Work out the finished part from the listing and answer in its coordinate system (mm). Give positions to 0.01 mm unless a question says otherwise; leave off trailing zeros. Loops run counter-clockwise (first coordinate to the right, second up) from the corner with the lowest first, then second, coordinate; pieces in that order, holes last. Notation, with made-up numbers: (38, 46) - (67, 46) arc R18 cw to (67, 68) - close; hole circle Ø5 at (37.5, 73). An arc over 180 degrees is marked (long way). Use CSV: the item, a comma, the result in double quotes.
from build123d import *

# Parameters (mm, degrees)
SKETCH1_R                                       = 2.4892
SKETCH1_R_2                                     = 2.5527
BOSS_EXTRUDE1_DEPTH                             = 3.175
FILLET1_R                                       = 4.7625
CSK_FOR_10_FLAT_HEAD_MACHINE_SCREW1_D           = 5.1054
CSK_FOR_10_FLAT_HEAD_MACHINE_SCREW1_DEPTH       = 19.05
CSK_FOR_10_FLAT_HEAD_MACHINE_SCREW1_CSINK_D     = 9.779
CSK_FOR_10_FLAT_HEAD_MACHINE_SCREW1_CSINK_ANGLE = 82
CSK_FOR_10_FLAT_HEAD_MACHINE_SCREW1_TIP         = 1.533816902


with BuildPart() as part:
    # Sketch1 → Boss-Extrude1 (new body)
    with BuildSketch(Plane.XY):
        Polygon((-37.846, 23.8125), (-37.846, -21.2725), (45.72, -21.2725), (45.72, 0.3175), (-21.59, 0.3175), (-21.59, 23.8125), align=None)
        with Locations((-29.845, -11.1125)):
            Circle(SKETCH1_R, mode=Mode.SUBTRACT)
        with Locations((-7.62, -11.1125)):
            Circle(SKETCH1_R, mode=Mode.SUBTRACT)
        with Locations((1.905, -11.1125)):
            Circle(SKETCH1_R_2, mode=Mode.SUBTRACT)
        with Locations((27.305, -11.1125)):
            Circle(SKETCH1_R_2, mode=Mode.SUBTRACT)
        with Locations((-29.845, 1.5875)):
            Circle(SKETCH1_R, mode=Mode.SUBTRACT)
        with Locations((-29.845, 14.2875)):
            Circle(SKETCH1_R, mode=Mode.SUBTRACT)
        with Locations((-29.845, -11.1125)):
            Circle(SKETCH1_R)
    extrude(amount=BOSS_EXTRUDE1_DEPTH)

    # Fillet1
    fillet1_edges = [part.edges().sort_by_distance(p)[0] for p in [
        (-37.846, 23.8125, 1.5875),
        (-21.59, 23.8125, 1.5875),
        (-21.59, 0.3175, 1.5875),
        (45.72, 0.3175, 1.5875),
        (45.72, -21.2725, 1.5875),
        (-37.846, -21.2725, 1.5875),
    ]]
    fillet(fillet1_edges, radius=FILLET1_R)

    # CSK for #10 Flat Head Machine Screw1
    with Locations(Plane.XY.offset(3.175)):
        with Locations((27.305, -11.1125)):
            CounterSinkHole(CSK_FOR_10_FLAT_HEAD_MACHINE_SCREW1_D / 2, CSK_FOR_10_FLAT_HEAD_MACHINE_SCREW1_CSINK_D / 2, depth=CSK_FOR_10_FLAT_HEAD_MACHINE_SCREW1_DEPTH, counter_sink_angle=CSK_FOR_10_FLAT_HEAD_MACHINE_SCREW1_CSINK_ANGLE)
            with Locations((0, 0, -(CSK_FOR_10_FLAT_HEAD_MACHINE_SCREW1_DEPTH + CSK_FOR_10_FLAT_HEAD_MACHINE_SCREW1_TIP / 2))):  # 118° drill point
                Cone(0, CSK_FOR_10_FLAT_HEAD_MACHINE_SCREW1_D / 2, CSK_FOR_10_FLAT_HEAD_MACHINE_SCREW1_TIP, mode=Mode.SUBTRACT)


solid = part.part
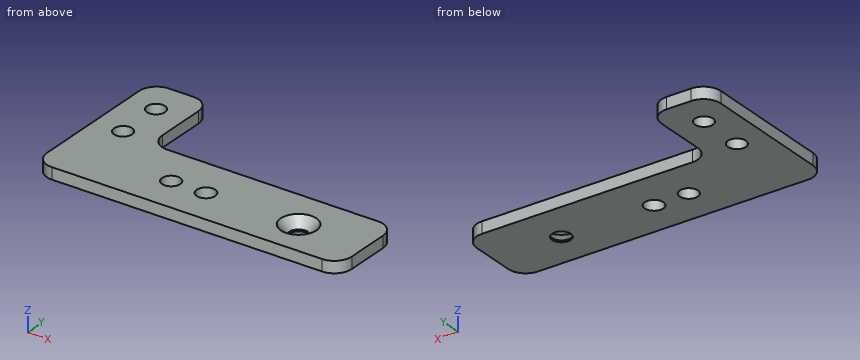
Item 1: Find the intervals of material crossed by line 1 (Y direction, x = 26, z = 0.8); line 2 (Y direction, x = -28, z = 0.6); line 3 (X direction, y = 9, z = 2.3), in increasing order.
Determined:
line 1,"y = -21.27 to -13.62, -8.61 to 0.32"
line 2,"y = -21.27 to -0.08, 3.26 to 12.62, 15.96 to 23.81"
line 3,"x = -37.85 to -21.59"
Item 2: A cutting plane is placed at C-C on x = -30.5. Determine the outline of the cut face in (y, z) (1 decimal), and give its area (3 significant figures).
Determined:
outline,"(-21.3, 0) - (-0.8, 0) - (-0.8, 3.2) - (-21.3, 3.2) - close; (4, 0) - (11.9, 0) - (11.9, 3.2) - (4, 3.2) - close; (16.7, 0) - (23.8, 0) - (23.8, 3.2) - (16.7, 3.2) - close"
area,"113 mm²"
Item 3: A cutting plane is placed at B-B on y = 2.5. Determine the outline of the cut face in (x, z) (3 decimals), and give its area (3 significant figures).
Determined:
outline,"(-37.846, 0) - (-32.161, 0) - (-32.161, 3.175) - (-37.846, 3.175) - close; (-27.529, 0) - (-20.831, 0) - (-20.831, 3.175) - (-27.529, 3.175) - close"
area,"39.3 mm²"
Item 4: A cutting plane is placed at A-A on x = -7.62. Determine the outline of the cut face in (y, z) (1 decimal), and give its area (3 significant figures).
Determined:
outline,"(-21.3, 0) - (-13.6, 0) - (-13.6, 3.2) - (-21.3, 3.2) - close; (-8.6, 0) - (0.3, 0) - (0.3, 3.2) - (-8.6, 3.2) - close"
area,"52.7 mm²"
Item 5: A cutting plane is placed at D-D on z = 2. State how many separate pieces and enclosed holes the cut face has, and give its area (3 significant figures).
Determined:
separate pieces,"1"
enclosed holes,"5"
area,"2,040 mm²"
Item 6: Given P1, Ø1, axis at y = 15, z = 2, coming from the +X side, flat-ended and moving along its own axis, determine where the tip first touches the part or whether it passes through.
Determined:
P1,"stops at x = -21.59"
